Geometry: final body of the model. Coordinates: model frame, mm. A direction names the side the tool comes from. Give positions to 0.01 mm unless a question says otherwise; leave off trailing zeros. Loops run counter-clockwise (first coordinate to the right, second up) from the corner with the lowest first, then second, coordinate; pieces in that order, holes last. Notation, with made-up numbers: (-27, 62) -> (-15, 62) arc R20 ccw to (-15, 75) -> close; hole circle Ø10 at (49.5, 38). An arc over 180 degrees is marked (long way). One line per item, written item: value. Start each with the question number.
Autodesk Inventor part; units mm, degrees
ref_plane "YZ Plane" through (0, 0, 0) normal (1, 0, 0) x (0, 1, 0)
ref_plane "XZ Plane" through (0, 0, 0) normal (0, 1, 0) x (-1, 0, 0)
ref_plane "XY Plane" through (0, 0, 0) normal (0, 0, 1) x (1, 0, 0)
sketch "bottom" plane through (0, 0, 0) normal (0, 1, 0) x (-1, 0, 0)
  line L0 (53.8137, 54.0949) -> (-46.1863, 54.0949)
  line L1 (-46.1863, 54.0949) -> (-46.1863, -65.9051)
  line L2 (-46.1863, -65.9051) -> (53.8137, -65.9051)
  line L3 (53.8137, -65.9051) -> (53.8137, 54.0949)
  line L4 (102.7933, -5.9051) -> (-137.2052, -5.9051)
  point P0 (0, 0)
  point P1 (53.8137, -5.9051)
  dimension "d0" = 120
  dimension "d1" = 100
extrude "Выдавливание1" add sketch "bottom" along normal blind 40
sketch "tube" plane through (-53.8137, 0, 54.0949) normal (0, 0, 1) x (1, 0, 0)
  circle A0 centre (51.5912, 40) radius 30
  line L0 (51.5912, 113.4013) -> (51.5912, -34.7388)
  line L1 (0, 40) -> (100, 40)
  point P0 (53.8137, 0)
  dimension "d6" = 60
extrude "Углубление 1" cut sketch "tube" against normal blind 120
sketch "paz1" plane through (-53.8137, 0, 54.0949) normal (0, 0, 1) x (1, 0, 0)
  line L0 (0, 0) -> (100, 0)
  line L1 (-0.0635, 15) -> (9.9365, 15)
  line L2 (9.9365, 15) -> (9.9365, 25)
  line L3 (9.9365, 25) -> (-0.0635, 25)
  line L4 (-0.0635, 25) -> (-0.0635, 15)
  line L5 (0, 40) -> (21.5912, 40)
  line L6 (89.6996, 15) -> (99.6996, 15)
  line L7 (99.6996, 15) -> (99.6996, 25)
  line L8 (99.6996, 25) -> (89.6996, 25)
  line L9 (89.6996, 25) -> (89.6996, 15)
  point P0 (53.8137, 0)
  dimension "d11" = 10
  dimension "d12" = 10
  dimension "d13" = 15
  dimension "d14" = 15
  dimension "d15" = 40
  dimension "d16" = 10
  dimension "d17" = 10
  dimension "d18" = 15
extrude "Паз 1" cut sketch "paz1" against normal up to next contours L4 L3 L2 L1
sketch "paz2" plane through (-53.8137, 0, 54.0949) normal (0, 0, 1) x (1, 0, 0)
  line L0 (0, 0) -> (100, 0)
  line L1 (0, 15) -> (10, 15)
  line L2 (10, 15) -> (10, 25)
  line L3 (10, 25) -> (0, 25)
  line L4 (0, 25) -> (0, 15)
  line L5 (0, 40) -> (21.5912, 40)
  line L6 (50, 55.3447) -> (50, -18.8311)
  line L7 (100, 15) -> (90, 15)
  line L8 (90, 15) -> (90, 25)
  line L9 (90, 25) -> (100, 25)
  line L10 (100, 25) -> (100, 15)
  line L11 (-10.5586, 20) -> (107.965, 20)
  line L12 (100, 0) -> (100, 40)
  arc A0 (21.5912, 40) -> (81.5912, 40) centre (51.5912, 40) ccw
  line L13 (81.5912, 40) -> (100, 40)
  line L14 (100, 25) -> (100, 40)
  line L15 (100, 15) -> (100, 0)
  line L16 (0, 25) -> (0, 40)
  line L17 (0, 40) -> (0, 25)
  line L18 (0, 0) -> (100, 0)
  line L19 (0, 15) -> (0, 0)
  point P0 (53.8137, 0)
  point P1 (53.8137, 0)
  point P2 (50, 0)
  point P3 (100, 20)
  point P4 (100, 15)
  dimension "d21" = 10
  dimension "d22" = 10
  dimension "d23" = 15
  dimension "d24" = 15
  dimension "d25" = 40
ref_plane "фронт1" through (-53.8137, 0, 44.0949) normal (0, 0, 1) x (1, 0, 0)
ref_plane "фронт2" through (46.1863, 0, -55.9051) normal (0, 0, -1) x (-1, 0, 0)
sketch "front_arc" plane through (-53.8137, 0, 44.0949) normal (0, 0, 1) x (1, 0, 0)
  arc A0 (21.5912, 40) -> (81.5912, 40) centre (51.5912, 40) ccw
  arc A1 (81.5912, 40) -> (21.5912, 40) centre (51.5912, 40) ccw
  line L0 (0, 40) -> (21.5912, 40)
  line L1 (81.5912, 40) -> (100, 40)
  line L2 (11.5912, 40) -> (21.5912, 40)
  line L3 (81.5912, 40) -> (91.5912, 40)
  line L4 (31.5912, 90) -> (31.5912, 74.641)
  line L5 (31.5912, 90) -> (51.5912, 90)
  line L6 (51.5912, 105.7627) -> (51.5912, 37.5467)
  line L7 (71.5912, 90) -> (71.5912, 74.641)
  line L8 (71.5912, 90) -> (51.5912, 90)
  arc A2 (91.5912, 40) -> (71.5912, 74.641) centre (51.5912, 40) ccw
  arc A3 (31.5912, 74.641) -> (11.5912, 40) centre (51.5912, 40) ccw
  point P0 (53.8137, 0)
  point P1 (31.5912, 40)
  point P2 (31.5912, 62.3607)
  point P3 (71.5912, 62.3607)
  dimension "d75" = 50
  dimension "d76" = 20
  dimension "d77" = 20
  dimension "d92" = 50
extrude "Выдавливание9" add sketch "front_arc" against normal blind 100 contours L0 A3 L4 L5 L6 A1 | A1 L6 L8 L7 A2 L1
sketch "top" plane through (-22.2225, 90, 44.0949) normal (0, 1, 0) x (1, 0, 0)
  line L0 (40, 0) -> (0, 0)
  line L1 (40, 0) -> (40, 100)
  line L2 (0, 100) -> (40, 100)
  line L3 (0, 0) -> (0, 100)
  line L4 (10, 0) -> (30, 0)
  line L5 (-37.6485, 50) -> (83.4602, 50)
  circle A0 centre (20, 50) radius 15
  line L6 (0, 100) -> (40, 100)
  line L7 (10, 20) -> (10, 0)
  line L8 (40, 0) -> (0, 0)
  line L9 (10, 20) -> (30, 20)
  line L10 (30, 20) -> (30, 0)
  line L11 (10, 100) -> (30, 100)
  line L12 (10, 80) -> (10, 100)
  line L13 (10, 80) -> (30, 80)
  line L14 (30, 80) -> (30, 100)
  line L15 (20, -16.8031) -> (20, 112.4511)
  point P0 (22.2225, 44.0949)
  point P1 (20, 0)
  point P2 (20, 100)
  point P3 (20, 100)
  dimension "d81" = 30
  dimension "d83" = 20
  dimension "d84" = 20
  dimension "d87" = 20
extrude "Выдавливание10" cut sketch "top" against normal blind 30 contours L0 L15 L9 L10 | L0 L7 L9 L15 | L14 L13 L15 L2 | L15 L13 L12 L2
extrude "Выдавливание11" cut sketch "top" against normal blind 25 contours A0 L15 L5 | L5 L15 A0 | L15 A0 L5 | L5 A0 L15
extrude "Выдавливание12" cut sketch "paz2" against normal blind 120 contours L7 L8 L11 L10 | L11 L8 L9 L10
equation "\"Радиус_гибки\" = Толщина"
equation "\"Ширина_просечки\" = Толщина"
equation "\"Глубина_просечки\" = 0.5 * Толщина"
equation "\"Размер_просечки\" = 4 * Толщина"
equation "\"Мин_остаток\" = 2 * Толщина"
equation "\"Радиус_перехода\" = Радиус_гибки"
equation "\"Радиус_Якоби\" = Толщина"
equation "\"Размер_зазора\" = Толщина"
properties part number "lw_3_ползунок"
Item 1: Section D-D, the plane z = 20.5. Output: boundary loops of the cut face in (x, y), then the cut area to 3 significant figures.
Item 2: Mould query, pull axis Y, two halves, no side actions, for faces 1 (the face through (11.621, 13.385, -5.065)), 2 (the face through (-2, 79, -35.905)), 3 (the face through (-43.877, 20, -5)), 4 (the face through (-16, 90, 6)). Classes: pulls with the +Y half, pulls with the -Y half, needs draft (parallel to the pull), parting line crosses it, or undercut.
Item 3: Access query for faces 5 (the face through (11.634, 78.158, -0.16)), 6 (the face through (-27, 65, 44.095)), 7 (the face through (17.778, 82, -5)), 8 (the face through (-2, 79, 24.095)). Directions: +Z, -Z, +X, -X, +Y, -Y. A direction counts if a zero-diameter tool reaches every point of the face in a straight line with its end or side. Return the directions, or none.
Item 4: Pin query (flat end, axial travel): pin 1 (18 mm diameter, centred on x = -2.22, z = -5.91, fed in from -Y); pin 2 (16 mm diameter, centred on x = -6, y = 83, fed in from +Z); pin 3 (8 mm diameter, centred on x = 42, z = 5, fed in from +Y); pin 4 (10 mm diameter, centred on y = 83, z = -44, fed in from +X). Return the tip coordinate at first contact, or that it passes through.
Item 5: Section A-A, the plane y = 20. Output: boundary loops of the cut face in (x, z), then the cut area to 3 significant figures.
Item 6: Section B-B, the plane z = -52. Output: boundary loops of the cut face in (x, y), then the cut area to 3 significant figures.
Item 7: Ray query, line 1 along Y through (x, z) = (-49.5, -28); line 2 along X through (y, z) = (79.5, -50); line 3 along Y through (x, z) = (-15.5, -33). Return the intervals inside material, ascending. Write a range as [from, to].
Item 8: Section C-C, the plane x = -19.5. Output: boundary loops of the cut face in (y, z).
Geometry check:
1. outline: (-53.81, 0) -> (46.19, 0) -> (46.19, 15) -> (36.19, 15) -> (36.19, 25) -> (46.19, 25) -> (46.19, 40) -> (37.78, 40) arc R40 ccw to (17.78, 74.64) -> (17.78, 90) -> (-22.22, 90) -> (-22.22, 74.64) arc R40 ccw to (-42.22, 40) -> (-53.81, 40) -> (-53.81, 25) -> (-43.88, 25) -> (-43.88, 15) -> (-53.81, 15) -> close; hole circle Ø60 at (-2.22, 40)
1. area: 3,960 mm2
2. face 1: undercut
2. face 2: needs draft
2. face 3: undercut
2. face 4: pulls with the +Y half
3. face 5: +Y
3. face 6: +Z, +X, -X, +Y
3. face 7: +Z, -Z, +X, +Y
3. face 8: +Z, +Y
4. pin 1: stops at y = 0
4. pin 2: stops at z = 44.09
4. pin 3: stops at y = 40
4. pin 4: stops at x = 17.78
5. outline: (-43.88, -65.91) -> (-24.58, -65.91) -> (-24.58, 54.09) -> (-43.88, 54.09) -> close; (20.14, -65.91) -> (36.19, -65.91) -> (36.19, 54.09) -> (20.14, 54.09) -> close
5. area: 4,240 mm2
6. outline: (-53.81, 0) -> (46.19, 0) -> (46.19, 15) -> (36.19, 15) -> (36.19, 25) -> (46.19, 25) -> (46.19, 40) -> (37.78, 40) arc R40 ccw to (17.78, 74.64) -> (17.78, 90) -> (7.78, 90) -> (7.78, 68.28) arc R30 cw (long way) to (-12.22, 68.28) -> (-12.22, 90) -> (-22.22, 90) -> (-22.22, 74.64) arc R40 ccw to (-42.22, 40) -> (-53.81, 40) -> (-53.81, 25) -> (-43.88, 25) -> (-43.88, 15) -> (-53.81, 15) -> close
6. area: 3,540 mm2
7. line 1: y = [0, 15], [25, 40]
7. line 2: x = [-22.22, -12.22], [7.78, 17.78]
7. line 3: y = [0, 13.1], [66.9, 90]
8. outline: (0, -65.91) -> (15.47, -65.91) -> (15.47, 54.09) -> (0, 54.09) -> close; (64.53, -55.91) -> (90, -55.91) -> (90, 44.09) -> (64.53, 44.09) -> close
